from build123d import *

# Parameters (mm, degrees)
SKETCH1_R           = 7.5
SKETCH1_R_2         = 5.1
BOSS_EXTRUDE1_DEPTH = 28.3
SKETCH4_R           = 27.5
BOSS_EXTRUDE3_DEPTH = 22
FILLET1_R           = 2
SKETCH5_R           = 2.125
CUT_EXTRUDE2_DEPTH  = 20
BOSS_EXTRUDE4_DEPTH = 20
SKETCH7_R           = 1.6
CUT_EXTRUDE3_DEPTH  = 15


with BuildPart() as part:
    # Sketch1 → Boss-Extrude1 (new body)
    with BuildSketch(Plane.XY):
        Circle(SKETCH1_R)
        Circle(SKETCH1_R_2, mode=Mode.SUBTRACT)
    extrude(amount=BOSS_EXTRUDE1_DEPTH)

    # Sketch4 → Boss-Extrude3 (add)
    with BuildSketch(Plane(origin=(0, 0, 0), x_dir=(-1, 0, 0), z_dir=(0, 0, -1))):
        Circle(SKETCH4_R)
    extrude(amount=BOSS_EXTRUDE3_DEPTH)

    # Fillet1
    fillet1_edges = [part.edges().sort_by_distance(p)[0] for p in [
        (-7.5, 0, 0),
    ]]
    fillet(fillet1_edges, radius=FILLET1_R)

    # Sketch5 → Cut-Extrude2 (cut)
    with BuildSketch(Plane(origin=(0, 0, -22), x_dir=(-1, 0, 0), z_dir=(0, 0, -1))):
        with Locations((0, 12)):
            Circle(SKETCH5_R)
        with Locations((12, 0)):
            Circle(SKETCH5_R)
        with Locations((0, -12)):
            Circle(SKETCH5_R)
        with Locations((-12, 0)):
            Circle(SKETCH5_R)
    extrude(amount=-CUT_EXTRUDE2_DEPTH, mode=Mode.SUBTRACT)

    # Sketch6 → Boss-Extrude4 (add)
    with BuildSketch(Plane.XY):
        with BuildLine():
            ThreePointArc((3.163858404, 4), (0, 5.1), (-3.163858404, 4))
            Line((-3.163858404, 4), (3.163858404, 4))
        make_face()
    extrude(amount=BOSS_EXTRUDE4_DEPTH)

    # Sketch7 → Cut-Extrude3 (cut)
    with BuildSketch(Plane(origin=(0, 0, 0), x_dir=(1, 0, 0), z_dir=(0, 1, 0))):
        with Locations(Location((0, -14, 0), (0, 0, 90))):
            Circle(SKETCH7_R)
    extrude(amount=CUT_EXTRUDE3_DEPTH, mode=Mode.SUBTRACT)


solid = part.part
Input: part model. Units: mm. Frame: model coordinates. A direction names the side the tool comes from. Give positions to 0.01 mm unless a question says otherwise; leave off trailing zeros. Loops run counter-clockwise (first coordinate to the right, second up) from the corner with the lowest first, then second, coordinate; pieces in that order, holes last. Notation, with made-up numbers: (2.25, -18.75) -> (13.25, -18.75) arc R17 ccw to (13.25, 1.25) -> close; hole circle Ø9 at (-20, 55.25). An arc over 180 degrees is marked (long way). Answer as a JSON object with one key per item and string values. Group by question number.
Item 1: Cut plane A-A, the plane x = 0. Return the cut outline in (y, z) (3 decimals).
Item 2: Reachability of faces 1 (the flat face through (0, 4, 10)), 2 (the cylindrical face through (13.6, 1.4, -12.1)), 3 (the cylindrical face through (-0.07, 5.73, 15.6)) from +Z, -Z, +X, -X, +Y, -Y: full face, straight path, thin tool, end or side. Return the list, or none.
Item 3: Cut plane B-B, the plane y = 0. Return the cut outline in (x, z) (3 decimals), and give its area (3 significant figures).
Item 4: Pull-direction query (X, two-part tool) for faces 4 (the flat face through (0, 0, -22)), 5 (the cylindrical face through (-1.63, -7.32, 14.97)), 6 (the cylindrical face through (-1, -5, 14)); classes: released by +X, released by -X, zero draft, split by the parting line, or undercut.
Item 5: Cut plane D-D, the plane z = 8.5. Return the cut outline in (x, y), and give its area (3 significant figures).
Item 6: Cut plane C-C, the plane z = -4. Return the cut outline in (x, y) (3 decimals), and give its area (3 significant figures).
Item 7: Pin query (flat end, axial travel): P1, Ø1.5, axis at x = 9.5, z = -11.5, coming from the +Y side; P2, Ø8, axis at y = 6, z = 3, coming from the +X side; P3, Ø8, axis at x = 14.5, y = -15, coming from the +Z side. Return the tip coordinate at first contact, or that it passes through.
Item 8: Line query: probe 1 along Y at (x, z) = (-1, -4.5) (3 decimals); probe 2 along Z at (x, y) = (-16, -3); probe 3 along Y at (x, z) = (-12, -7) (3 decimals). Output: solid intervals per line, ascending.
Checks:
{
 "1": {"outline": "(-27.5, -22) -> (-14.125, -22) -> (-14.125, -2) -> (-9.875, -2) -> (-9.875, -22) -> (9.875, -22) -> (9.875, -2) -> (14.125, -2) -> (14.125, -22) -> (27.5, -22) -> (27.5, 0) -> (9.5, 0) arc R2 cw to (7.5, 2) -> (7.5, 12.4) -> (4, 12.4) -> (4, 0) -> (-5.1, 0) -> (-5.1, 28.3) -> (-7.5, 28.3) -> (-7.5, 2) arc R2 cw to (-9.5, 0) -> (-27.5, 0) -> close; (4, 15.6) -> (7.5, 15.6) -> (7.5, 28.3) -> (5.1, 28.3) -> (5.1, 20) -> (4, 20) -> close"},
 "2": {"face 1": "+Z", "face 2": "-Z", "face 3": "+Y"},
 "3": {"outline": "(-27.5, -22) -> (-14.125, -22) -> (-14.125, -2) -> (-9.875, -2) -> (-9.875, -22) -> (9.875, -22) -> (9.875, -2) -> (14.125, -2) -> (14.125, -22) -> (27.5, -22) -> (27.5, 0) -> (9.5, 0) arc R2 cw to (7.5, 2) -> (7.5, 28.3) -> (5.1, 28.3) -> (5.1, 0) -> (-5.1, 0) -> (-5.1, 28.3) -> (-7.5, 28.3) -> (-7.5, 2) arc R2 cw to (-9.5, 0) -> (-27.5, 0) -> close", "area": "1,180 mm²"},
 "4": {"face 4": "zero draft", "face 5": "split by the parting line", "face 6": "undercut"},
 "5": {"outline": "circle Ø15 at (0, 0); hole (-3.16, 4) arc R5.1 ccw (long way) to (3.16, 4) -> close", "area": "99.8 mm²"},
 "6": {"outline": "circle Ø55 at (0, 0); hole circle Ø4.25 at (-12, 0); hole circle Ø4.25 at (0, -12); hole circle Ø4.25 at (0, 12); hole circle Ø4.25 at (12, 0)", "area": "2,320 mm²"},
 "7": {"P1": "stops at y = 26.07", "P2": "stops at x = 27.29", "P3": "stops at z = 0"},
 "8": {"probe 1": "y = -27.482 to -13.875, -10.125 to 10.125, 13.875 to 27.482", "probe 2": "z = -22 to 0", "probe 3": "y = -24.744 to -2.125, 2.125 to 24.744"}
}
